```python
from build123d import *

# Parameters (mm, degrees)
SKETCH1_R           = 7
BOSS_EXTRUDE1_DEPTH = 2
SKETCH2_R           = 5.95
BOSS_EXTRUDE2_DEPTH = 7
SKETCH3_R           = 3.5
CUT_EXTRUDE1_DEPTH  = 1.8
CHAMFER1_SIZE       = 1


with BuildPart() as part:
    # Sketch1 → Boss-Extrude1 (new body)
    with BuildSketch(Plane(origin=(0, 0, 0), x_dir=(1, 0, 0), z_dir=(0, 1, 0))):
        with Locations(Location((0, 0, 0), (0, 0, 270))):
            Circle(SKETCH1_R)
    extrude(amount=BOSS_EXTRUDE1_DEPTH)

    # Sketch2 → Boss-Extrude2 (add)
    with BuildSketch(Plane(origin=(0, 2, 0), x_dir=(1, 0, 0), z_dir=(0, 1, 0))):
        with Locations(Location((0, 0, 0), (0, 0, 270))):
            Circle(SKETCH2_R)
    extrude(amount=BOSS_EXTRUDE2_DEPTH)

    # Sketch3 → Cut-Extrude1 (cut)
    with BuildSketch(Plane.XZ):
        with Locations(Location((0, 0, 0), (0, 0, 270))):
            Circle(SKETCH3_R)
    extrude(amount=-CUT_EXTRUDE1_DEPTH, mode=Mode.SUBTRACT)

    # Chamfer1
    chamfer1_edges = [part.edges().sort_by_distance(p)[0] for p in [
        (0, 9, -5.95),
    ]]
    chamfer(chamfer1_edges, length=CHAMFER1_SIZE)


solid = part.part
```
For this review, take the finished solid that the model builds, in its own axes (mm). A direction names the side the tool comes from. Coordinates: 2 decimals unless noted, no trailing zeros. Write each loop counter-clockwise with the first axis right and the second up, starting at its lowest first coordinate (ties: lowest second). Pieces come first, ordered by that corner, then holes. Notation, with made-up numbers: (-40, -23) - (12, -23) arc R31 cw to (12, 6) - close; hole circle Ø6 at (75, 1). An arc over 180 degrees is marked (long way). Answer in a Markdown table with one row per item. Add a question column.
Q1. Draft analysis for pull direction Z (two halves, no side actions). For faces 1 (the flat face through (0, 9, 0)), 2 (the flat face through (0, 1.8, 0)), 3 (the cylindrical face through (-6.834, 0.986, -1.517)), state which applies: +Z half, -Z half, draft (parallel to the pull), parting line (faces both ways), or undercut.
Q2. We need section C-C, the plane y = 7.5. State the section outline as (x, z) points.
Q3. For P1, Ø3, axis at y = 1, z = 5.5, coming from the -X side; P2, Ø1, axis at x = -0.5, y = 3.5, coming from the -Z side; P3, Ø3.5, axis at x = 1, z = -1, coming from the -Y side, all flat-tipped, find the tip position at first contact; note any pin that passes through.
Q4. We need section B-B, the plane x = 0. State the section outline as (y, z) points.
Q5. For probe 1 along X at (y, z) = (1.4, 0); probe 2 along Y at (x, z) = (0.5, 0); probe 3 along Y at (x, z) = (3.5, 6), list the stretches that pass through material, from the lowest coordinate up.
Q6. We need section A-A, the plane z = 0. State the section outline as (x, y) points, and give its area (3 significant figures).
Q7. Tool access review of faces 4 (the cylindrical face through (-3.417, 0.887, 0.759)), 5 (the flat face through (-6, 2, -2)), 6 (the flat face through (-3, 0, 3)): name each direction out of +Z, -Z, +X, -X, +Y, -Y from which nothing blocks a thin tool from reaching the whole face with its end or side.
Answer list:
| question | item | result |
|---|---|---|
| 1 | face 1 | draft |
| 1 | face 2 | undercut |
| 1 | face 3 | parting line |
| 2 | outline | circle Ø11.9 at (0, 0) |
| 3 | P1 | stops at x = -5.74 |
| 3 | P2 | stops at z = -5.95 |
| 3 | P3 | stops at y = 1.8 |
| 4 | outline | (0, -7) - (2, -7) - (2, -5.95) - (8, -5.95) - (9, -4.95) - (9, 4.95) - (8, 5.95) - (2, 5.95) - (2, 7) - (0, 7) - (0, 3.5) - (1.8, 3.5) - (1.8, -3.5) - (0, -3.5) - close |
| 5 | probe 1 | x = -7 to -3.5, 3.5 to 7 |
| 5 | probe 2 | y = 1.8 to 9 |
| 5 | probe 3 | y = 0 to 2 |
| 6 | outline | (-7, 0) - (-3.5, 0) - (-3.5, 1.8) - (3.5, 1.8) - (3.5, 0) - (7, 0) - (7, 2) - (5.95, 2) - (5.95, 8) - (4.95, 9) - (-4.95, 9) - (-5.95, 8) - (-5.95, 2) - (-7, 2) - close |
| 6 | area | 97.7 mm2 |
| 7 | face 4 | -Y |
| 7 | face 5 | +Y |
| 7 | face 6 | +Z, -Z, +X, -X, -Y |
